Print and shaded views of the part. All mm, measured from the part's lowest x, y and z. A direction names the side the tool comes from. Give positions to 0.01 mm unless a question says otherwise; leave off trailing zeros. Write each loop counter-clockwise with the first axis right and the second up, starting at its lowest first coordinate (ties: lowest second). Pieces come first, ordered by that corner, then holes. Notation, with made-up numbers: (-1, 36.25) -> (37, 36.25) arc R20 ccw to (37, 50.25) -> close; hole circle Ø6 at (64, -35). An arc over 180 degrees is marked (long way). Put each result on its own line as item: value.
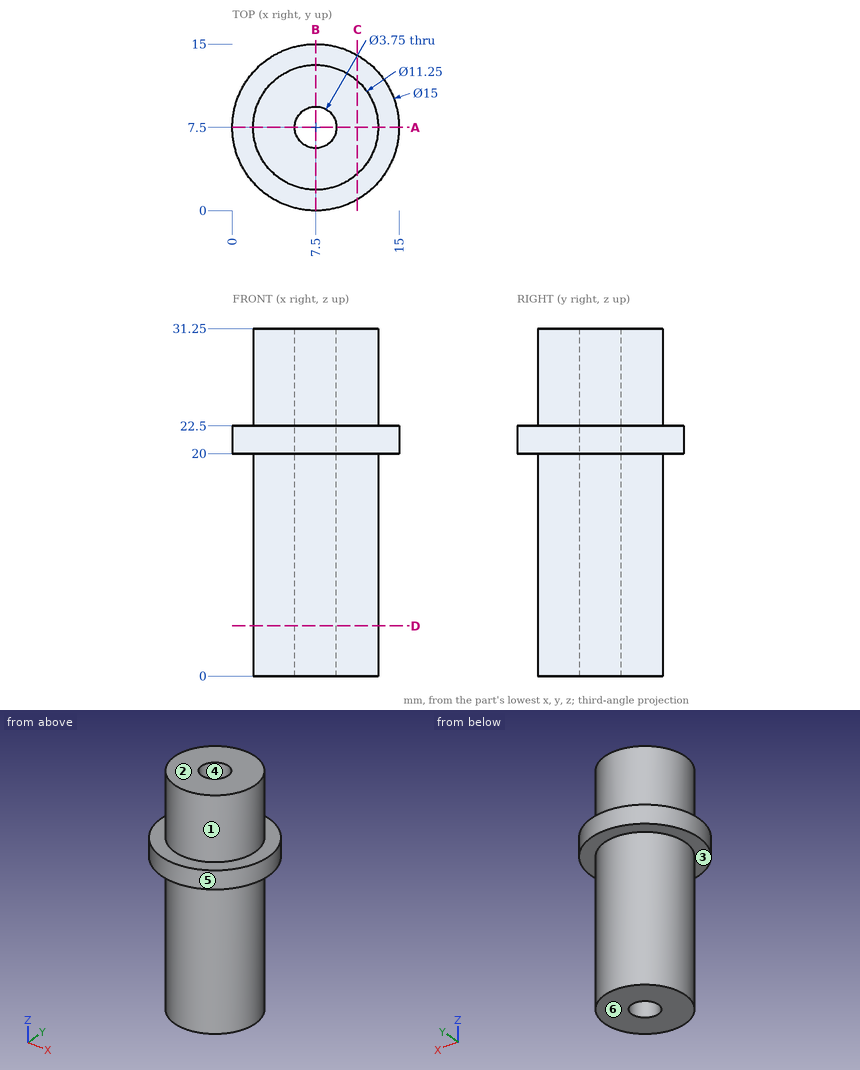
1) Slice it at D-D (z = 4.5). Write the cut outline in (x, y) (3 decimals), plus the area to 3 significant figures.
Filled sheet:
outline: circle Ø11.25 at (7.5, 7.5); hole circle Ø3.75 at (7.5, 7.5)
area: 88.4 mm2
2) Slice it at A-A (y = 7.5). Write the cut outline in (x, z) (3 decimals).
Filled sheet:
outline: (0, 20) -> (1.875, 20) -> (1.875, 0) -> (5.625, 0) -> (5.625, 31.25) -> (1.875, 31.25) -> (1.875, 22.5) -> (0, 22.5) -> close; (9.375, 0) -> (13.125, 0) -> (13.125, 20) -> (15, 20) -> (15, 22.5) -> (13.125, 22.5) -> (13.125, 31.25) -> (9.375, 31.25) -> close
3) Pin check, flat tips, straight feed: pin 1 (1 mm diameter, centred on x = 9.5, z = 10.5, fed in from -Y); pin 2 (6 mm diameter, centred on x = 10.5, z = 17.5, fed in from +Y); pin 3 (4 mm diameter, centred on x = 5, y = 7.5, fed in from -Z); pin 4 (5 mm diameter, centred on x = 9.5, z = 12, fed in from -Y) (3 decimals). Stop position of each tip, or through.
Filled sheet:
pin 1: y = 2.08
pin 2: y = 14.88
pin 3: z = 0
pin 4: y = 1.875
4) Slice it at C-C (x = 11.25). Write the cut outline in (y, z).
Filled sheet:
outline: (1, 20) -> (3.31, 20) -> (3.31, 0) -> (11.69, 0) -> (11.69, 20) -> (14, 20) -> (14, 22.5) -> (11.69, 22.5) -> (11.69, 31.25) -> (3.31, 31.25) -> (3.31, 22.5) -> (1, 22.5) -> close
5) Tool access for the marked faces 1, 2 and 3: list every direction of +Z, -Z, +X, -X, +Y, -Y with a clear straight run to the whole face (end or side of a thin tool).
Filled sheet:
face 1: +Z
face 2: +Z, +X, -X, +Y, -Y
face 3: -Z
6) Wall check: L1, parallel to Y at x = 7.5, z = 12 (3 decimals); L2, parallel to Y at x = 7.5, z = 22 (3 decimals); L3, parallel to Z at x = 2, y = 10.25. Give the ranges that are in metal, low to high.
Filled sheet:
L1: 1.875 to 5.625, 9.375 to 13.125
L2: 0 to 5.625, 9.375 to 15
L3: 20 to 22.5
7) Pull direction Y, two halves, no side cores. Call the marked faces 4, 5 and 6: released by +Y, released by -Y, zero draft, split by the parting line, or undercut.
Filled sheet:
face 4: undercut
face 5: split by the parting line
face 6: zero draft
